```python
from build123d import *

# Parameters (mm, degrees)
SKETCH1_W           = 22
SKETCH1_H           = 12
BOSS_EXTRUDE1_DEPTH = 22
SKETCH2_W           = 32
SKETCH2_H           = 2
BOSS_EXTRUDE2_DEPTH = 12
SKETCH3_R           = 1
CUT_EXTRUDE1_DEPTH  = 22
SKETCH5_R           = 6
BOSS_EXTRUDE3_DEPTH = 5


with BuildPart() as part:
    # Sketch1 → Boss-Extrude1 (new body)
    with BuildSketch(Plane(origin=(0, 0, 0), x_dir=(1, 0, 0), z_dir=(0, 1, 0))):
        with Locations((11, 6)):
            Rectangle(SKETCH1_W, SKETCH1_H)
    extrude(amount=BOSS_EXTRUDE1_DEPTH)

    # Sketch2 → Boss-Extrude2 (add, through all)
    with BuildSketch(Plane.XY):
        with Locations((11, 17)):
            Rectangle(SKETCH2_W, SKETCH2_H)
    extrude(amount=-BOSS_EXTRUDE2_DEPTH)

    # Sketch3 → Cut-Extrude1 (cut)
    with BuildSketch(Plane(origin=(0, 18, 0), x_dir=(1, 0, 0), z_dir=(0, 1, 0))):
        with Locations((-2.5, 6)):
            Circle(SKETCH3_R)
        with Locations((24.5, 6)):
            Circle(SKETCH3_R)
    extrude(amount=-CUT_EXTRUDE1_DEPTH, mode=Mode.SUBTRACT)

    # Sketch5 → Boss-Extrude3 (add)
    with BuildSketch(Plane(origin=(0, 22, 0), x_dir=(1, 0, 0), z_dir=(0, 1, 0))):
        with Locations((16, 6)):
            Circle(SKETCH5_R)
    extrude(amount=BOSS_EXTRUDE3_DEPTH)


solid = part.part
```
Source: CAD feature listing. Evaluate the final solid. Frame: model axes, mm. A direction names the side the tool comes from. Round coordinates to 2 decimals unless told otherwise and drop trailing zeros. Write each loop counter-clockwise with the first axis right and the second up, starting at its lowest first coordinate (ties: lowest second). Pieces come first, ordered by that corner, then holes. Notation, with made-up numbers: M -28,42.25 L 13,42.25 A29 cw 13,78.25 Z; hole C -32,-31 d6. An arc over 180 degrees is marked long. Answer as a JSON object with one key per item and string values. Group by question number.
(1) Section query D-D on x = 21. Output: boundary loops of the cut face in (y, z).
(2) Section query B-B on z = -5.5. State how many separate pieces and enclosed holes the cut face has, then the cut area to 3 significant figures.
(3) Ray query, line 1 (X direction, y = 16.8, z = -6); line 2 (Z direction, x = -2.5, y = 16.7); line 3 (Y direction, x = 11, z = -9.75). Return the intervals inside material, ascending. Write a range as [from, to].
(4) Mould query, pull axis X, two halves, no side actions, for faces 1 (the flat face through (0, 20, -6)), 2 (the cylindrical face through (-2.63, 17.01, -6.99)), 3 (the flat face through (22, 8, -6)). Classes: +X half, -X half, draft (parallel to the pull), parting line (faces both ways), or undercut.
(5) Section query A-A on x = 24.5. Output: boundary loops of the cut face in (y, z).
(6) First-contact query: pin 1 (6 mm diameter, centred on x = 3, z = -10, fed in from +Y); pin 2 (2.5 mm diameter, centred on x = -2, z = -4, fed in from -Y); pin 3 (1.5 mm diameter, centred on y = 5.5, z = -8, fed in from -X). Flat tips, straight axial feed; report the tip coordinate or a pass-through.
(7) Section query C-C on z = -1.25. Output: boundary loops of the cut face in (x, y).
(8) Reachability of faces 4 (the flat face through (21, 22, -11)), 5 (the flat face through (-1, 18, -6)), 6 (the flat face through (21, 22, -1)) from +Z, -Z, +X, -X, +Y, -Y: full face, straight path, thin tool, end or side. Return the list, or none.
Computed values:
{
 "1": {"outline": "M 0,-12 L 22,-12 L 22,-9.32 L 27,-9.32 L 27,-2.68 L 22,-2.68 L 22,0 L 0,0 Z"},
 "2": {"separate pieces": "3", "enclosed holes": "0", "area": "557 mm^2"},
 "3": {"line 1": "[-5, -3.5], [-1.5, 23.5], [25.5, 27]", "line 2": "[-12, -7], [-5, 0]", "line 3": "[0, 22]"},
 "4": {"face 1": "-X half", "face 2": "undercut", "face 3": "+X half"},
 "5": {"outline": "M 16,-12 L 18,-12 L 18,-7 L 16,-7 Z; M 16,-5 L 18,-5 L 18,0 L 16,0 Z"},
 "6": {"pin 1": "y = 22", "pin 2": "y = 16", "pin 3": "x = 0"},
 "7": {"outline": "M -5,16 L 0,16 L 0,0 L 22,0 L 22,16 L 27,16 L 27,18 L 22,18 L 22,22 L 19.67,22 L 19.67,27 L 12.33,27 L 12.33,22 L 0,22 L 0,18 L -5,18 Z"},
 "8": {"face 4": "-Z, +X, +Y", "face 5": "+Z, -Z, -X, +Y", "face 6": "+Z, +X, +Y"}
}
